from build123d import *

# Parameters (mm, degrees)
BOSS_EXTRUDE1_DEPTH = 20
CUT_EXTRUDE1_DEPTH  = 20
SKETCH4_R           = 4
SKETCH4_R_2         = 2
CUT_EXTRUDE2_DEPTH  = 37


with BuildPart() as part:
    # Sketch1 → Boss-Extrude1 (new body)
    with BuildSketch(Plane.XY):
        with BuildLine():
            Line((-40, 0), (-60, 0))
            Line((-60, 0), (-60, 5))
            Line((-60, 5), (-54.083269132, 5))
            ThreePointArc((-54.083269132, 5), (-50.885258387, 6.156469426), (-49.166608302, 9.090909091))
            ThreePointArc((-49.166608302, 9.090909091), (-31.980107453, 38.435305739), (0, 50))
            Line((0, 50), (0, 40))
            ThreePointArc((0, 40), (-28.284271247, 28.284271247), (-40, 0))
        make_face()
    boss_extrude1 = extrude(amount=BOSS_EXTRUDE1_DEPTH)

    # Sketch2 → Cut-Extrude1 (cut)
    with BuildSketch(Plane.XZ):
        with BuildLine():
            ThreePointArc((-48, 10), (-49.234633135, 11.847759065), (-51.414213562, 11.414213562))
            Line((-51.414213562, 11.414213562), (-48.585786438, 8.585786438))
            ThreePointArc((-48.585786438, 8.585786438), (-48.152240935, 9.234633135), (-48, 10))
        make_face()
        with BuildLine():
            Line((-48.585786438, 8.585786438), (-51.414213562, 11.414213562))
            ThreePointArc((-51.414213562, 11.414213562), (-51.414213562, 8.585786438), (-48.585786438, 8.585786438))
        make_face()
    cut_extrude1 = extrude(amount=-CUT_EXTRUDE1_DEPTH, mode=Mode.SUBTRACT)

    # Sketch4 → Cut-Extrude2 (cut)
    with BuildSketch(Plane(origin=(0, 5, 0), x_dir=(1, 0, 0), z_dir=(0, 1, 0))):
        with Locations((-50, -10)):
            Circle(SKETCH4_R)
        with Locations((-50, -10)):
            Circle(SKETCH4_R_2, mode=Mode.SUBTRACT)
    cut_extrude2 = extrude(amount=CUT_EXTRUDE2_DEPTH, mode=Mode.SUBTRACT)

    # Mirror1: Boss-Extrude1, Cut-Extrude1, Cut-Extrude2 across plane
    add(boss_extrude1.mirror(Plane(origin=(0, 0, 20), x_dir=(0, 0, 1), z_dir=(1, 0, 0))))
    add(cut_extrude1.mirror(Plane(origin=(0, 0, 20), x_dir=(0, 0, 1), z_dir=(1, 0, 0))), mode=Mode.SUBTRACT)
    add(cut_extrude2.mirror(Plane(origin=(0, 0, 20), x_dir=(0, 0, 1), z_dir=(1, 0, 0))), mode=Mode.SUBTRACT)


solid = part.part
Could you check a few things on this model? Use its own coordinates, in mm. A direction names the side the tool comes from. Give positions to 0.01 mm unless a question says otherwise; leave off trailing zeros. Order: outer loops, then holes, each group sorted by start corner. A loop starts at its lowest first (then second) coordinate and runs counter-clockwise, first axis right, second up.
Item 1: If we section it at D-D, the plane x = -44.5: Write out the boundary of the cut face in (y, z), plus the area to 3 significant figures.
Item 2: If we section it at A-A, the plane y = 7: Write out the boundary of the cut face in (x, z), plus the area to 3 significant figures.
Item 3: I need wall thicknesses on line 1 (X direction, y = 35, z = 9.25); line 2 (X direction, y = 11.5, z = 10); line 3 (Y direction, x = -55, z = 11.5). Which ranges of each line are inside material? Lowest first, please.
Item 4: I'm going to push flat-ended pins straight in: pin 1 (1.5 mm diameter, centred on y = 42.5, z = 11.5, fed in from -X); pin 2 (10 mm diameter, centred on x = -18.5, y = 32, fed in from +Z); pin 3 (5 mm diameter, centred on x = -50, z = 10, fed in from +Y); pin 4 (12 mm diameter, centred on y = 37.5, z = 4, fed in from -X). Where does each tip first touch, or does it pass through?
Item 5: If we mould it in two halves opening along X, with no side actions, what happens to faces 1 (the face through (52, 5, 11)), 2 (the face through (-5, 40, 20)), 3 (the face through (53.75, 5.01, 7.64))? For each: pulls with the +X half, pulls with the -X half, needs draft (parallel to the pull), parting line crosses it, or undercut.
Item 6: For faces 4 (the face through (-52, 5, 11)), 5 (the face through (57, 5, 10)), 6 (the face through (-57, 5, 10)), 7 (the face through (-60, 2, 10)), which set-ups out of +Z, -Z, +X, -X, +Y, -Y let a thin tool reach every point of the face, with its end or its side?
Item 7: If we section it at B-B, the plane z = 16.25: Write out the boundary of the cut face in (x, y), plus the area to 3 significant figures.
Item 8: If we section it at C-C, the plane y = 28: Write out the boundary of the cut face in (x, z), plus the area to 3 significant figures.
Values:
1. outline: (0, 0) - (22.8, 0) - (22.8, 20) - (0, 20) - close
1. area: 456 mm2
2. outline: (-50.08, 0) - (-39.38, 0) - (-39.38, 20) - (-50.08, 20) - (-50.08, 14) arc R4 cw (long way) to (-50.08, 6) - close; (39.38, 0) - (50.08, 0) - (50.08, 6) arc R4 cw (long way) to (50.08, 14) - (50.08, 20) - (39.38, 20) - close
2. area: 376 mm2
3. line 1: x = -35.71 to -19.36, 19.36 to 35.71
3. line 2: x = -46 to -38.31, 38.31 to 46
3. line 3: y = 0 to 5
4. pin 1: stops at x = -27.51
4. pin 2: stops at z = 20
4. pin 3: stops at y = 5
4. pin 4: stops at x = -38.83
5. face 1: undercut
5. face 2: needs draft
5. face 3: pulls with the +X half
6. face 4: +Y
6. face 5: +Z, -Z, +X, +Y
6. face 6: +Z, -Z, -X, +Y
6. face 7: +Z, -Z, -X, +Y, -Y
7. outline: (-60, 0) - (-40, 0) arc R40 cw to (40, 0) - (60, 0) - (60, 5) - (54.08, 5) arc R5 cw to (49.17, 9.09) arc R50 ccw to (-49.17, 9.09) arc R5 cw to (-54.08, 5) - (-60, 5) - close
7. area: 1,520 mm2
8. outline: (-41.42, 0) - (-28.57, 0) - (-28.57, 20) - (-41.42, 20) - close; (28.57, 0) - (41.42, 0) - (41.42, 20) - (28.57, 20) - close
8. area: 514 mm2
